```python
from build123d import *

# Parameters (mm, degrees)
F0_R     = 3
F1_DEPTH = 38.5
F0_R_2   = 14
F2_DEPTH = 24.5
F3_SIZE  = 2
F5_R     = 22
F5_R_2   = 6.35
F6_DEPTH = 7.3
F7_DEPTH = 3.1


with BuildPart() as f1:
    # F0 (on Top) → F1 (new body)
    with BuildSketch(Plane.XY):
        Circle(F0_R)
    extrude(amount=F1_DEPTH)

    # F0 (on Top) → F2 (join)
    with BuildSketch(Plane.XY):
        Circle(F0_R_2)
        Circle(F0_R, mode=Mode.SUBTRACT)
    extrude(amount=F2_DEPTH)

    # F3
    f3_edges = [f1.edges().sort_by_distance(p)[0] for p in [
        (-14, 0, 0),
        (-14, 0, 24.5),
        (-3, 0, 38.5),
    ]]
    chamfer(f3_edges, length=F3_SIZE)

    # F5 (on offset) → F6 (join)
    with BuildSketch(Plane.XY.offset(29.6)):
        Circle(F5_R)
        Circle(F5_R_2, mode=Mode.SUBTRACT)
        Circle(F5_R_2)
    extrude(amount=F6_DEPTH)

    # F5 (on offset) → F7 (join)
    with BuildSketch(Plane.XY.offset(29.6)):
        Circle(F5_R_2)
    extrude(amount=-F7_DEPTH)


solid = f1.part
```
Check sheet for the modelled part. Datum: model origin and axes. Units: mm. A direction names the side the tool comes from. Give positions to 0.01 mm unless a question says otherwise; leave off trailing zeros. Loops run counter-clockwise (first coordinate to the right, second up) from the corner with the lowest first, then second, coordinate; pieces in that order, holes last. Notation, with made-up numbers: M 26,58.5 L 65,58.5 A23 ccw 65,81.5 Z; hole C 48,51 d9. An arc over 180 degrees is marked long. Answer as CSV lines item,"result".
Item 1: Sectioned sample at A-A, the plane x = 0. Enter the section's corners in (y, z), then the cut area to 3 significant figures.
Reply:
outline,"M -22,29.6 L -6.35,29.6 L -6.35,26.5 L -3,26.5 L -3,24.5 L -12,24.5 L -14,22.5 L -14,2 L -12,0 L 12,0 L 14,2 L 14,22.5 L 12,24.5 L 3,24.5 L 3,26.5 L 6.35,26.5 L 6.35,29.6 L 22,29.6 L 22,36.9 L 2.6,36.9 L 1,38.5 L -1,38.5 L -2.6,36.9 L -22,36.9 Z"
area,"1,060 mm^2"
Item 2: Sectioned sample at D-D, the plane z = 27.5. Enter the section's corners in (x, y).
Reply:
outline,"C 0,0 d12.7"
Item 3: Sectioned sample at C-C, the plane z = 18.5. Enter the section's corners in (x, y), then the cut area to 3 significant figures.
Reply:
outline,"C 0,0 d28"
area,"616 mm^2"
Item 4: Scan lines: L1, parallel to Z at x = -4, y = -9; L2, parallel to Z at x = -9.5, y = 18; L3, parallel to Z at x = 12, y = 3. Record each from-to range of solid material in increasing order.
Reply:
L1,"0 to 24.5, 29.6 to 36.9"
L2,"29.6 to 36.9"
L3,"0.37 to 24.13, 29.6 to 36.9"
Item 5: Set-up check for faces 4 (the face through (12.932, -5.362, 12.106)), 5 (the face through (-4.769, -21.477, 33.199)), 6 (the face through (-3, 0, 25)): record each of +Z, -Z, +X, -X, +Y, -Y from which the full face is reachable in a straight line by a thin tool's end or side.
Reply:
face 4,"-Z"
face 5,"+Z, -Z"
face 6,"none"
Item 6: Depth check by flat-ended pin: pin 1 Ø8 at (y, z) = (8.5, 10) entering from +X; pin 2 Ø6 at (x, z) = (4.5, 31) entering from +Y; pin 3 Ø1.5 at (x, y) = (5.5, -2) entering from +Z. Enter the tip coordinate at first touch or a pass-through.
Reply:
pin 1,"x = 13.26"
pin 2,"y = 21.95"
pin 3,"z = 36.9"
Item 7: Draft check along Z on faces 1 (the face through (5, -5, 29.6)), 2 (the face through (0, 0, 0)), 3 (the face through (0, 0, 38.5)). Enter one of: pulls with the +Z half, pulls with the -Z half, needs draft (parallel to the pull), parting line crosses it, or undercut.
Reply:
face 1,"undercut"
face 2,"pulls with the -Z half"
face 3,"pulls with the +Z half"
